Read the model definition and answer for the solid it produces. Units are mm, in the model's axes. A direction names the side the tool comes from. Round coordinates to 2 decimals unless told otherwise and drop trailing zeros. Loops run counter-clockwise (first coordinate to the right, second up) from the corner with the lowest first, then second, coordinate; pieces in that order, holes last. Notation, with made-up numbers: (40, 7.5) -> (90, 7.5) arc R21 cw to (90, 39.5) -> close; hole circle Ø7 at (42.25, -2.5). An arc over 180 degrees is marked (long way). Put each result on its own line as item: value.
from build123d import *

# Parameters (mm, degrees)
F0_W     = 12.1401943831
F0_H     = 2
F1_DEPTH = 25
F4_DEPTH = 5.1
F8_R     = 1.99999


# Not quite as in the source:
# - a fillet or chamfer is up to 0.001 mm smaller than in the source, because OpenCascade refuses the exact size


with BuildPart() as f1:
    # F0 (on Front) → F1 (new body)
    with BuildSketch(Plane.XZ):
        with BuildLine():
            Line((-1.75, 1.75), (-13.8901943831, 1.75))
            ThreePointArc((-13.8901943831, 1.75), (-12.3581823788, -6.5783986115), (-6.3047601065, -12.5))
            Line((-6.3047601065, -12.5), (6.3047601065, -12.5))
            ThreePointArc((6.3047601065, -12.5), (12.3581823788, -6.5783986115), (13.8901943831, 1.75))
            Line((13.8901943831, 1.75), (1.75, 1.75))
            Line((1.75, 1.75), (1.75, 0))
            ThreePointArc((1.75, 0), (0, -1.75), (-1.75, 0))
            Line((-1.75, 0), (-1.75, 1.75))
        make_face()
        with Locations((7.8200971915, 2.75)):
            Rectangle(F0_W, F0_H)
        with Locations((-7.8200971915, 2.75)):
            Rectangle(F0_W, F0_H)
    extrude(amount=F1_DEPTH)

    # F3 (on face) → F4 (cut)
    with BuildSketch(Plane(origin=(0, 0, 0), x_dir=(-1, 0, 0), z_dir=(0, 1, 0))):
        with BuildLine():
            ThreePointArc((-10.3942291681, 3.75), (-1.9034531373, -10.8848227433), (11.05, 0))
            ThreePointArc((11.05, 0), (10.8848227433, 1.9034531373), (10.3942291681, 3.75))
            Line((10.3942291681, 3.75), (7.9056941504, 3.75))
            ThreePointArc((7.9056941504, 3.75), (8.5363143047, 1.921936027), (8.75, 0))
            ThreePointArc((8.75, 0), (-1.921936027, -8.5363143047), (-7.9056941504, 3.75))
            Line((-7.9056941504, 3.75), (-10.3942291681, 3.75))
        make_face()
    extrude(amount=-F4_DEPTH, mode=Mode.SUBTRACT)

    # F7: F1 across face


with BuildPart() as f1_1:
    add(f1.part)
    add(f1.part.mirror(Plane(origin=(0, -25, -3.8986050214), x_dir=(1, 0, 0), z_dir=(0, -1, 0))))

    # F8 (radius 2 in the source; OpenCascade refuses exactly that, so slightly less here)
    f8_edges = [f1_1.edges().sort_by_distance(p)[0] for p in [
        (13.890194, -25, 3.75),
        (-13.890194, -25, 3.75),
    ]]
    fillet(f8_edges, radius=F8_R)


solid = f1_1.part
Item 1: Which of the six approach directions +Z, -Z, +X, -X, +Y, -Y give full straight-line access (tool end or side, diameter ignored) to faces 5 (the flat face through (0, -50, -2)), 6 (the flat face through (-1, -44.9, -9)), 7 (the flat face through (-1.75, -25, 2))?
Derived:
face 5: +Z, -Z, +X, -X, -Y
face 6: -Y
face 7: +Z, +Y, -Y
Item 2: Find the intervals of material crossed by line 1 along Z through (x, y) = (0, -46.4); line 2 along X through (y, z) = (-5, -6.25); line 3 along Y through (x, z) = (3.75, -8), in increasing order.
Derived:
line 1: z = -12.5 to -11.05, -8.75 to -1.75
line 2: x = -12.53 to -9.11, -6.12 to 6.12, 9.11 to 12.53
line 3: y = -44.9 to -5.1
Item 3: The part is cut by section B-B (x = 0). Determine the outline of the cut face in (y, z).
Derived:
outline: (-50, -12.5) -> (0, -12.5) -> (0, -11.05) -> (-5.1, -11.05) -> (-5.1, -8.75) -> (0, -8.75) -> (0, -1.75) -> (-50, -1.75) -> (-50, -8.75) -> (-44.9, -8.75) -> (-44.9, -11.05) -> (-50, -11.05) -> close
Item 4: Flat-ended cylindrical pins translate along their axes: pin 1 Ø1.1 at (y, z) = (-18.5, 1.5) entering from +X; pin 2 Ø1 at (y, z) = (-44, -9.5) entering from +X; pin 3 Ø6 at (y, z) = (-38, -9) entering from -X. Find the tip coordinate at first contact, or state that the pin passes through.
Derived:
pin 1: stops at x = 13.97
pin 2: stops at x = 10.72
pin 3: stops at x = -12.65
Item 5: The part is cut by section D-D (z = -4.75). Determine the outline of the cut face in (x, y).
Derived:
outline: (-13.17, -50) -> (-9.98, -50) -> (-9.98, -44.9) -> (-7.35, -44.9) -> (-7.35, -50) -> (7.35, -50) -> (7.35, -44.9) -> (9.98, -44.9) -> (9.98, -50) -> (13.17, -50) -> (13.17, 0) -> (9.98, 0) -> (9.98, -5.1) -> (7.35, -5.1) -> (7.35, 0) -> (-7.35, 0) -> (-7.35, -5.1) -> (-9.98, -5.1) -> (-9.98, 0) -> (-13.17, 0) -> close
Item 6: The part is cut by section A-A (z = -0.5). Determine the outline of the cut face in (x, y), then the cut area to 3 significant figures.
Derived:
outline: (-13.99, -50) -> (-11.04, -50) -> (-11.04, -44.9) -> (-8.74, -44.9) -> (-8.74, -50) -> (-1.68, -50) -> (-1.68, 0) -> (-8.74, 0) -> (-8.74, -5.1) -> (-11.04, -5.1) -> (-11.04, 0) -> (-13.99, 0) -> close; (1.68, -50) -> (8.74, -50) -> (8.74, -44.9) -> (11.04, -44.9) -> (11.04, -50) -> (13.99, -50) -> (13.99, 0) -> (11.04, 0) -> (11.04, -5.1) -> (8.74, -5.1) -> (8.74, 0) -> (1.68, 0) -> close
area: 1,180 mm^2
Item 7: For a pull along Z with two mould halves and no side action, classify faces 1 (the flat face through (0, -25, -12.5)), 2 (the flat face through (-1, -5.1, -9)), 3 (the cylindrical face through (-13.29, -24.65, 3.18)), 4 (the flat face through (1.75, -25, 2)) as pulls with the +Z half, pulls with the -Z half, needs draft (parallel to the pull), parting line crosses it, or undercut.
Derived:
face 1: pulls with the -Z half
face 2: undercut
face 3: pulls with the +Z half
face 4: needs draft
